The listing builds one solid part. Answer for the finished solid, in the listing's coordinates (mm). A direction names the side the tool comes from. Give positions to 0.01 mm unless a question says otherwise; leave off trailing zeros. Loops run counter-clockwise (first coordinate to the right, second up) from the corner with the lowest first, then second, coordinate; pieces in that order, holes last. Notation, with made-up numbers: M 4.5,61 L 9.5,61 A32 cw 9.5,87 Z; hole C -11.5,55.5 d3. An arc over 180 degrees is marked long. Use one line per item in the form item = value. Start each with the question number.
1. The part is cut by section B-B (y = -0.25). Write down the section's boundary in (x, z), and give its area (3 significant figures).
2. The mould has two halves that part along Y. Classify faces 3 (the face through (1.179, 0.543, 2.004)), 4 (the face through (0, -4.64, 0)), 5 (the face through (-1.01, 2.26, -0.65)): released by +Y, released by -Y, zero draft, split by the parting line, or undercut.
3. The part is cut by section A-A (z = 0). Write down the section's boundary in (x, y) (3 decimals), and give its area (3 significant figures).
4. The part is cut by section C-C (y = 2). Write down the section's boundary in (x, z), and give its area (3 significant figures).
5. Straight lines are drawn through the part: line 1 (Z direction, x = 0.05, y = 2.5); line 2 (Y direction, x = 1.9, z = -0.2); line 3 (X direction, y = -1, z = -0.05). For each, find the intervals that lie inside material, in ascending order. Write a range as from..to.
6. For faces 1 (the face through (1, 0, 1)), 2 (the face through (1.15, 0.54, -2.02)), determine the directions among +Z, -Z, +X, -X, +Y, -Y from which every point of the face is accessible in a straight line to the end or side of a thin tool.
7. This flat-tipped pin is pushed along its axis until it touches: pin 1 Ø1 at (x, z) = (-1.5, -1) entering from +Y. Where does it stop, or does it pass through?
from build123d import *

# Parameters (mm, degrees)
SKETCH2_OUTSIDE_W   = 13.154
SKETCH2_OUTSIDE_H   = 13.154
CUT_EXTRUDE1_DEPTH  = 9.580601773
SKETCH3_R           = 1.1303
BOSS_EXTRUDE1_DEPTH = 4.64


with BuildPart() as part:
    # Sketch1 → Revolve1 (revolve)
    with BuildSketch(Plane.XY, mode=Mode.PRIVATE) as revolve1_sk:
        with BuildLine():
            Line((4.231088913, 0), (1.2, 1.75))
            Line((1.2, 1.75), (1.2, 2.75))
            ThreePointArc((1.2, 2.75), (2.099622467, 4.433550528), (1.26447926, 6.15))
            Line((1.26447926, 6.15), (0, 6.15))
            Line((0, 6.15), (0, 0))
            Line((0, 0), (4.231088913, 0))
        make_face()
    revolve(revolve1_sk.sketch.rotate(Axis((0, 0, 0), (0, 1, 0)), 90), axis=Axis((0, 0, 0), (0, 1, 0)))

    # Sketch2 outside → Cut-Extrude1 (cut, through all)
    with BuildSketch(Plane.XZ):
        Rectangle(SKETCH2_OUTSIDE_W, SKETCH2_OUTSIDE_H)
        Polygon((0, 2.684678752), (-2.325, 1.342339376), (-2.325, -1.342339376), (0, -2.684678752), (2.325, -1.342339376), (2.325, 1.342339376), align=None, mode=Mode.SUBTRACT)
    extrude(amount=-CUT_EXTRUDE1_DEPTH, mode=Mode.SUBTRACT)

    # Sketch3 → Boss-Extrude1 (add)
    with BuildSketch(Plane.XZ):
        with Locations(Location((0, 0, 0), (0, 0, 270))):
            Circle(SKETCH3_R)
    extrude(amount=BOSS_EXTRUDE1_DEPTH)


solid = part.part
Derived:
q1.outline = C 0,0 d2.26
q1.area = 4.01 mm2
q2.face_3 = zero draft
q2.face_4 = released by -Y
q2.face_5 = undercut
q3.outline = M -2.325,0 L -1.13,0 L -1.13,-4.64 L 1.13,-4.64 L 1.13,0 L 2.325,0 L 2.325,1.1 L 1.2,1.75 L 1.2,2.75 A2.1 ccw 1.264,6.15 L -1.264,6.15 A2.1 ccw -1.2,2.75 L -1.2,1.75 L -2.325,1.1 Z
q3.area = 32.8 mm2
q4.outline = C 0,0 d2.4
q4.area = 4.52 mm2
q5.line_1 = -1.2..1.2
q5.line_2 = 0..1.34, 3.6..5.35
q5.line_3 = -1.13..1.13
q6.face_1 = -Y
q6.face_2 = -Z, +X, +Y, -Y
q7.pin_1 = 6.12
